```python
from build123d import *

# Parameters (mm, degrees)
BASE_FLANGE1_DEPTH            = 3
EDGE_FLANGE1_STRIP_W          = 20
EDGE_FLANGE1_STRIP_H          = 3
EDGE_FLANGE1_STRIP_CUT_DEPTH  = 40
EDGE_FLANGE1_RELIEF_W         = 21.5
EDGE_FLANGE1_RELIEF_H         = 1.5
EDGE_FLANGE1_RELIEF_CUT_DEPTH = 3
EDGE_FLANGE1_DEPTH            = 40
SKETCH10_R                    = 1.75
SKETCH10_R_2                  = 6
CUT_EXTRUDE1_DEPTH            = 226.971790275
EDGE_FLANGE2_STRIP_W          = 18
EDGE_FLANGE2_STRIP_H          = 3
EDGE_FLANGE2_STRIP_CUT_DEPTH  = 212
EDGE_FLANGE2_DEPTH            = 212
EDGE_FLANGE3_STRIP_W          = 18
EDGE_FLANGE3_STRIP_H          = 3
EDGE_FLANGE3_STRIP_CUT_DEPTH  = 212
EDGE_FLANGE3_DEPTH            = 212
MIRROR1_START                 = -107.5
MIRROR1_DEPTH                 = 213.5
MIRROR1_START_2               = 104.5
MIRROR1_2_DEPTH               = 1.5
MIRROR1_3_DEPTH               = 212
CUT_EXTRUDE2_DEPTH            = 10


# Read off the part's stored shape, not the designer's step: Mirror1
# Sheet-metal steps are written as plain solids
with BuildPart() as part:
    # Sketch1 → Base-Flange1 (new body)
    with BuildSketch(Plane(origin=(0, 0, 0), x_dir=(1, 0, 0), z_dir=(0, 1, 0))):
        Polygon((-107.5, -42.5), (108.5, -42.5), (108.5, -2.5), (107.5, -2.5), (107.5, 42.5), (-107.5, 42.5), align=None)
    extrude(amount=-BASE_FLANGE1_DEPTH)

    # Edge-Flange1 strip (across the edge) → Edge-Flange1 strip cut (cut)
    with BuildSketch(Plane(origin=(108.5, 0, 42.5), x_dir=(-1, 0, 0), z_dir=(0, 0, -1))):
        with Locations((-6, -1.5)):
            Rectangle(EDGE_FLANGE1_STRIP_W, EDGE_FLANGE1_STRIP_H)
    extrude(amount=EDGE_FLANGE1_STRIP_CUT_DEPTH, mode=Mode.SUBTRACT)

    # Edge-Flange1 relief (on the sheet) → Edge-Flange1 relief cut (cut)
    with BuildSketch(Plane(origin=(104.5, 0, 42.5), x_dir=(-1, 0, 0), z_dir=(0, 1, 0))):
        with Locations((-9.25, -40.75)):
            Rectangle(EDGE_FLANGE1_RELIEF_W, EDGE_FLANGE1_RELIEF_H)
    extrude(amount=-EDGE_FLANGE1_RELIEF_CUT_DEPTH, mode=Mode.SUBTRACT)

    # Edge-Flange1 section (across the edge) → Edge-Flange1 (add)
    with BuildSketch(Plane(origin=(108.5, 0, 42.5), x_dir=(-1, 0, 0), z_dir=(0, 0, -1))):
        with BuildLine():
            Line((-3, 4), (-3, 36))
            Line((-3, 36), (0, 36))
            Line((0, 36), (0, 4))
            ThreePointArc((0, 4), (1.171572875, 1.171572875), (4, 0))
            Line((4, 0), (4, -3))
            ThreePointArc((4, -3), (-0.949747468, -0.949747468), (-3, 4))
        make_face()
    extrude(amount=EDGE_FLANGE1_DEPTH)

    # Sketch10 → Cut-Extrude1 (cut, through all)
    with BuildSketch(Plane(origin=(111.5, 0, 0), x_dir=(0, 0, -1), z_dir=(1, 0, 0))):
        with Locations(Location((-38, 30, 0), (0, 0, 90))):
            Circle(SKETCH10_R)
        with Locations(Location((-7, 30, 0), (0, 0, 90))):
            Circle(SKETCH10_R)
        with Locations(Location((-22.5, 14.5, 0), (0, 0, 90))):
            Circle(SKETCH10_R_2)
    extrude(amount=-CUT_EXTRUDE1_DEPTH, mode=Mode.SUBTRACT)

    # Edge-Flange2 strip (across the edge) → Edge-Flange2 strip cut (cut)
    with BuildSketch(Plane(origin=(-107.5, 0, 42.5), x_dir=(0, 0, -1), z_dir=(1, 0, 0))):
        with Locations((-6, -1.5)):
            Rectangle(EDGE_FLANGE2_STRIP_W, EDGE_FLANGE2_STRIP_H)
    extrude(amount=EDGE_FLANGE2_STRIP_CUT_DEPTH, mode=Mode.SUBTRACT)

    # Edge-Flange2 section (across the edge) → Edge-Flange2 (add)
    with BuildSketch(Plane(origin=(-107.5, 0, 42.5), x_dir=(0, 0, -1), z_dir=(1, 0, 0))):
        with BuildLine():
            Line((-3, 3), (-3, 19.5))
            Line((-3, 19.5), (0, 19.5))
            Line((0, 19.5), (0, 3))
            ThreePointArc((0, 3), (0.878679656, 0.878679656), (3, 0))
            Line((3, 0), (3, -3))
            ThreePointArc((3, -3), (-1.242640687, -1.242640687), (-3, 3))
        make_face()
    extrude(amount=EDGE_FLANGE2_DEPTH)

    # Edge-Flange3 strip (across the edge) → Edge-Flange3 strip cut (cut)
    with BuildSketch(Plane(origin=(104.5, 19.5, 45.5), x_dir=(0, -1, 0), z_dir=(-1, 0, 0))):
        with Locations((-6, -1.5)):
            Rectangle(EDGE_FLANGE3_STRIP_W, EDGE_FLANGE3_STRIP_H)
    extrude(amount=EDGE_FLANGE3_STRIP_CUT_DEPTH, mode=Mode.SUBTRACT)

    # Edge-Flange3 section (across the edge) → Edge-Flange3 (add)
    with BuildSketch(Plane(origin=(104.5, 19.5, 45.5), x_dir=(0, -1, 0), z_dir=(-1, 0, 0))):
        with BuildLine():
            Line((-3, 3), (-3, 20))
            Line((-3, 20), (0, 20))
            Line((0, 20), (0, 3))
            ThreePointArc((0, 3), (0.878679656, 0.878679656), (3, 0))
            Line((3, 0), (3, -3))
            ThreePointArc((3, -3), (-1.242640687, -1.242640687), (-3, 3))
        make_face()
    extrude(amount=EDGE_FLANGE3_DEPTH)

    # Mirror1 outline → Mirror1 (cut)
    with BuildSketch(Plane.YZ.offset(MIRROR1_START)):
        with BuildLine():
            Line((-3, -42.5), (-2.196152423, -42.5))
            ThreePointArc((-2.196152423, -42.5), (-2.795554958, -41.052914271), (-3, -39.5))
            Line((-3, -39.5), (-3, -42.5))
        make_face()
    extrude(amount=MIRROR1_DEPTH, mode=Mode.SUBTRACT)

    # Mirror1 2 outline → Mirror1 2 (cut)
    with BuildSketch(Plane.YZ.offset(MIRROR1_START_2)):
        with BuildLine():
            ThreePointArc((-3, -39.5), (-2.795554958, -41.052914271), (-2.196152423, -42.5))
            Line((-2.196152423, -42.5), (0, -42.5))
            Line((0, -42.5), (0, -38))
            Line((0, -38), (-3, -38))
            Line((-3, -38), (-3, -39.5))
        make_face()
    extrude(amount=MIRROR1_2_DEPTH, mode=Mode.SUBTRACT)

    # Mirror1 3 outline → Mirror1 3 (add)
    with BuildSketch(Plane.YZ.offset(MIRROR1_START)):
        with BuildLine():
            Line((3, -45.5), (16.5, -45.5))
            ThreePointArc((16.5, -45.5), (18.621320344, -46.378679656), (19.5, -48.5))
            Line((19.5, -48.5), (19.5, -65.5))
            Line((19.5, -65.5), (22.5, -65.5))
            Line((22.5, -65.5), (22.5, -48.5))
            ThreePointArc((22.5, -48.5), (20.742640687, -44.257359313), (16.5, -42.5))
            Line((16.5, -42.5), (3, -42.5))
            ThreePointArc((3, -42.5), (0.878679656, -41.621320344), (0, -39.5))
            Line((0, -39.5), (0, -42.5))
            Line((0, -42.5), (-2.196152423, -42.5))
            ThreePointArc((-2.196152423, -42.5), (0, -44.696152423), (3, -45.5))
        make_face()
    extrude(amount=MIRROR1_3_DEPTH)

    # Sketch19 → Cut-Extrude2 (cut)
    with BuildSketch(Plane(origin=(0, 0, 0), x_dir=(1, 0, 0), z_dir=(0, 1, 0))):
        Polygon((107.5, -1), (107.5, 42.5), (106, 42.5), (104.5, 38), (104.5, -1), align=None)
    extrude(amount=-CUT_EXTRUDE2_DEPTH, mode=Mode.SUBTRACT)


solid = part.part
```
Could you check a few things on this model? Use its own coordinates, in mm. A direction names the side the tool comes from. Give positions to 0.01 mm unless a question says otherwise; leave off trailing zeros. Write each loop counter-clockwise with the first axis right and the second up, starting at its lowest first coordinate (ties: lowest second). Pieces come first, ordered by that corner, then holes. Notation, with made-up numbers: (36, -33) -> (83, -33) arc R26 cw to (83, -6) -> close; hole circle Ø7 at (61, 6.25). An arc over 180 degrees is marked (long way). Write each question's results on one line, items separated by ' | '.
1. I need wall thicknesses on L1, parallel to Z at x = 109, y = 30; L2, parallel to Z at x = 25.5, y = 8.5; L3, parallel to X at y = 3.5, z = 43. Which ranges of each line are inside material? Lowest first, please.
Check sheet entries:
L1: z = 2.5 to 5.25, 8.75 to 36.25, 39.75 to 42.5 | L2: z = -45.5 to -42.5, 42.5 to 45.5 | L3: x = -107.5 to 104.5
2. I want a section at B-B, the plane y = 25. Write out the boundary of the cut face in (x, z).
Check sheet entries:
outline: (108.5, 2.5) -> (111.5, 2.5) -> (111.5, 42.5) -> (108.5, 42.5) -> close
3. I want a section at C-C, the plane z = -15. Write out the boundary of the cut face in (x, y).
Check sheet entries:
outline: (-107.5, -3) -> (104.5, -3) -> (104.5, 0) -> (-107.5, 0) -> close
4. I want a section at A-A, the plane x = -34. Write out the boundary of the cut face in (y, z), then the cut area to 3 significant figures.
Check sheet entries:
outline: (-3, -39.5) arc R6 ccw to (3, -45.5) -> (16.5, -45.5) arc R3 cw to (19.5, -48.5) -> (19.5, -65.5) -> (22.5, -65.5) -> (22.5, -48.5) arc R6 ccw to (16.5, -42.5) -> (3, -42.5) arc R3 cw to (0, -39.5) -> (0, 39.5) arc R3 cw to (3, 42.5) -> (16.5, 42.5) arc R6 ccw to (22.5, 48.5) -> (22.5, 65.5) -> (19.5, 65.5) -> (19.5, 48.5) arc R3 cw to (16.5, 45.5) -> (3, 45.5) arc R6 ccw to (-3, 39.5) -> close | area: 505 mm²
5. Will these pins go through, and if not, where does the flat tip stop? pin 1 Ø8 at (y, z) = (30.5, 10.5) entering from -X; pin 2 Ø4 at (x, z) = (-7, -32) entering from +Y; pin 3 Ø7 at (x, y) = (29.5, 10) entering from +Z; pin 4 Ø7 at (y, z) = (14.5, 22.5) entering from -X.
Check sheet entries:
pin 1: stops at x = 108.5 | pin 2: stops at y = 0 | pin 3: stops at z = 45.5 | pin 4: passes through
6. On a 3-axis mill with a long thin cutter (end or side, diameter ignored), from which of +Z, -Z, +X, -X, +Y, -Y can I reach the whole of each face in a straight line? I mean faces 4 (the cylindrical face through (-2.984, -1.289, 43.696)), 5 (the flat face through (-3, 10, -42.5)), 6 (the flat face through (108.5, 24, 23)), 7 (the flat face through (-3, 0, -1)). Say none if no direction works.
Check sheet entries:
face 4: +Z, -X, -Y | face 5: +X, -X, +Y | face 6: +Z, -Z, -X, +Y | face 7: -X, +Y
7. If we mould it in two halves opening along Z, with no side actions, what happens to faces 1 (the flat face through (-3, 10, -45.5)), 2 (the flat face through (-3, 10, 42.5)), 3 (the flat face through (-3, -3, -1))? For each: released by +Z, released by -Z, zero draft, split by the parting line, or undercut.
Check sheet entries:
face 1: released by -Z | face 2: undercut | face 3: zero draft
